The model under review builds one solid part; all positions refer to its coordinate system, in mm. A direction names the side the tool comes from. Round coordinates to 2 decimals unless told otherwise and drop trailing zeros. Order: outer loops, then holes, each group sorted by start corner. A loop starts at its lowest first (then second) coordinate and runs counter-clockwise, first axis right, second up.
1) Machinability: for faces 5 (the face through (10, 3, 0)), 6 (the face through (-13.3, 0.5, -5)), 7 (the face through (4.379, 2, 0)), which of the approach directions +Z, -Z, +X, -X, +Y, -Y give a long, thin tool a straight path to every point of the face, cutting with its end or side? Answer none if there is none.
2) Consider section B-B (x = -11). Give the boundary of the cut face in (y, z).
3) Consider section A-A (z = -6.95). Give the boundary of the cut face in (x, y), then the cut area to 3 significant figures.
4) To check wall thickness, follow L1, parallel to X at y = 1.65, z = -1; L2, parallel to Z at x = -11, y = 0.65; L3, parallel to X at y = 0.45, z = 6.95. State the ranges of each line that lie inside material, in increasing order.
5) Consider section D-D (z = 0). Give the boundary of the cut face in (x, y).
6) Consider section C-C (y = 0.45). Give the boundary of the cut face in (x, z), then the cut area to 3 significant figures.
7) Clearance check with flat-ended pins moving along their axes: P1, Ø1.2, axis at x = 3.5, y = 2, coming from the -Z side; P2, Ø1.1, axis at y = 0.5, z = -5.5, coming from the +X side; P3, Ø0.6, axis at y = 1.5, z = 7, coming from the -X side. State where each tip first meets the part, or that it passes through.
8) Mouldability with a two-part tool opening along X and no side actions: class faces 1 (the face through (3, 2, -1.194)), 2 (the face through (15, 2, 0)), 3 (the face through (-11.6, 0.5, -3.3)), 4 (the face through (-14, 0.5, 6.9)) as pulls with the +X half, pulls with the -X half, needs draft (parallel to the pull), parting line crosses it, or undercut.
from build123d import *

# Parameters (mm, degrees)
SKETCH_1_W             = 28
SKETCH_1_H             = 17.5
EXTRUDE_1_DEPTH        = 1
EXTRUDE_START          = -1
SKETCH_2_W             = 5
SKETCH_2_H             = 9
EXTRUDE_2_DEPTH        = 4.5
FILLET_1_R             = 0.5
SKETCH_3_W             = 2.088904022
SKETCH_3_H             = 2.32763591
EXTRUDE_3_DEPTH        = 1.5
SKETCH_6_W             = 1.4
SKETCH_6_H             = 10
CUT_EXTRUDE_2_DEPTH    = 2
SKETCH_4_R             = 0.75
CUT_EXTRUDE_1_DEPTH    = 2
SKETCH_5_W             = 2
SKETCH_5_H             = 1
EXTRUDE_4_DEPTH        = 1.8
PATTERN_LINEAR_1_COUNT = 2
PATTERN_LINEAR_1_PITCH = 4.7


with BuildPart() as part:
    # 草图1 → 凸台-拉伸1 (new body)
    with BuildSketch(Plane(origin=(0, 0, 0), x_dir=(1, 0, 0), z_dir=(0, 1, 0))):
        Rectangle(SKETCH_1_W, SKETCH_1_H)
    extrude(amount=EXTRUDE_1_DEPTH)

    # 草图2 → 凸台-拉伸2 (add)
    with BuildSketch(Plane(origin=(0, 1, 0), x_dir=(1, 0, 0), z_dir=(0, 1, 0)).offset(EXTRUDE_START)):
        with Locations((12.5, 0)):
            Rectangle(SKETCH_2_W, SKETCH_2_H)
    extrude(amount=EXTRUDE_2_DEPTH)

    # 圆角1
    fillet_1_edges = [part.edges().sort_by_distance(p)[0] for p in [
        (12.5, 4.5, 4.5),
        (12.5, 4.5, -4.5),
    ]]
    fillet(fillet_1_edges, radius=FILLET_1_R)

    # 草图3 → 凸台-拉伸3 (add)
    with BuildSketch(Plane(origin=(0, 1, 0), x_dir=(1, 0, 0), z_dir=(0, 1, 0))):
        with Locations((3.334941172, 0.029841486)):
            Rectangle(SKETCH_3_W, SKETCH_3_H)
    extrude(amount=EXTRUDE_3_DEPTH)

    # 草图6 → 切除-拉伸2 (cut, through all)
    with BuildSketch(Plane(origin=(0, 1, 0), x_dir=(1, 0, 0), z_dir=(0, 1, 0))):
        with Locations((-13.3, 0)):
            Rectangle(SKETCH_6_W, SKETCH_6_H)
    extrude(amount=-CUT_EXTRUDE_2_DEPTH, mode=Mode.SUBTRACT)

    # 草图4 → 切除-拉伸1 (cut, through all)
    with BuildSketch(Plane(origin=(0, 1, 0), x_dir=(1, 0, 0), z_dir=(0, 1, 0))):
        with Locations((-11, 6.95)):
            Circle(SKETCH_4_R)
        with Locations((-11, 3.75)):
            Circle(SKETCH_4_R)
        with Locations((-11, -3.75)):
            Circle(SKETCH_4_R)
        with Locations((-11, -6.95)):
            Circle(SKETCH_4_R)
    extrude(amount=-CUT_EXTRUDE_1_DEPTH, mode=Mode.SUBTRACT)

    # 草图5 → 凸台-拉伸4 (add)
    with BuildSketch(Plane(origin=(0, 1, 0), x_dir=(1, 0, 0), z_dir=(0, 1, 0)).offset(EXTRUDE_START)):
        with Locations((5.2, -7.25)):
            Rectangle(SKETCH_5_W, SKETCH_5_H)
    extrude_4 = extrude(amount=EXTRUDE_4_DEPTH)

    # 阵列(线性)1: 凸台-拉伸4 ×2
    with Locations(*[(-i * PATTERN_LINEAR_1_PITCH, 0, 0) for i in range(1, PATTERN_LINEAR_1_COUNT)]):
        add(extrude_4)


solid = part.part
Answer below:
1. face 5: +Z, -Z, +Y
1. face 6: -X, +Y, -Y
1. face 7: -Z, +Y
2. outline: (0, -8.75) - (1, -8.75) - (1, -7.7) - (0, -7.7) - close; (0, -6.2) - (1, -6.2) - (1, -4.5) - (0, -4.5) - close; (0, -3) - (1, -3) - (1, 3) - (0, 3) - close; (0, 4.5) - (1, 4.5) - (1, 6.2) - (0, 6.2) - close; (0, 7.7) - (1, 7.7) - (1, 8.75) - (0, 8.75) - close
3. outline: (-14, 0) - (-11.75, 0) - (-11.75, 1) - (-14, 1) - close; (-10.25, 0) - (14, 0) - (14, 1) - (-10.25, 1) - close
3. area: 26.5 mm2
4. L1: x = 2.29 to 4.38, 10 to 15
4. L2: z = -8.75 to -7.7, -6.2 to -4.5, -3 to 3, 4.5 to 6.2, 7.7 to 8.75
4. L3: x = -14 to -11.75, -10.25 to 14
5. outline: (-12.6, 0) - (15, 0) - (15, 4.5) - (10, 4.5) - (10, 1) - (4.38, 1) - (4.38, 2.5) - (2.29, 2.5) - (2.29, 1) - (-12.6, 1) - close
6. outline: (-14, -8.75) - (14, -8.75) - (14, -4.5) - (15, -4.5) - (15, 4.5) - (14, 4.5) - (14, 8.75) - (-14, 8.75) - (-14, 5) - (-12.6, 5) - (-12.6, -5) - (-14, -5) - close; hole circle Ø1.5 at (-11, -6.95); hole circle Ø1.5 at (-11, -3.75); hole circle Ø1.5 at (-11, 3.75); hole circle Ø1.5 at (-11, 6.95)
6. area: 478 mm2
7. P1: stops at z = -1.19
7. P2: stops at x = 14
7. P3: stops at x = -0.5
8. face 1: needs draft
8. face 2: pulls with the +X half
8. face 3: undercut
8. face 4: pulls with the -X half
